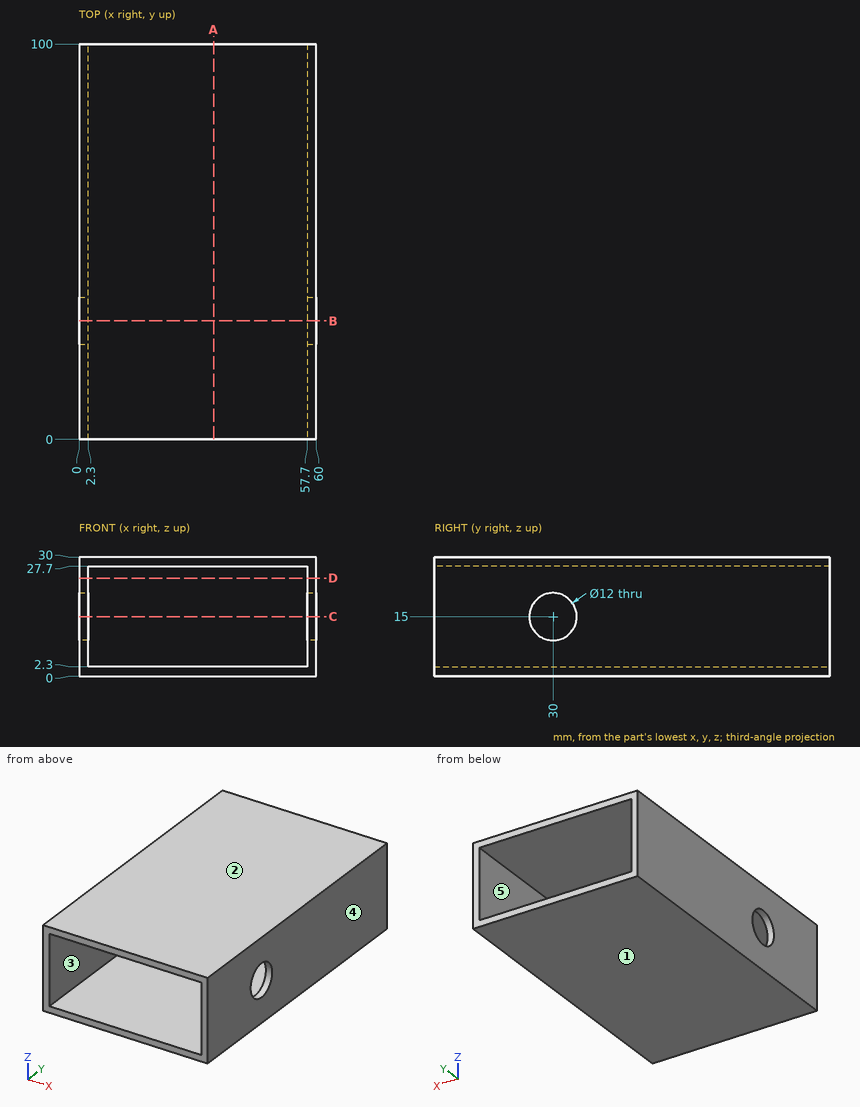
Check sheet for the drawn part. Datum: minimum x, y, z corner. Units: mm. A direction names the side the tool comes from. Coordinates: 2 decimals unless noted, no trailing zeros. Write each loop counter-clockwise with the first axis right and the second up, starting at its lowest first coordinate (ties: lowest second). Pieces come first, ordered by that corner, then holes. Notation, with made-up numbers: M 23,32.5 L 77,32.5 A33 cw 77,71.5 Z; hole C -21,27.5 d6. An arc over 180 degrees is marked long. One line per item, written item: value.
Item 1: Scan lines: line 1 along Z through (x, y) = (34, 49); line 2 along Y through (x, z) = (59, 15); line 3 along X through (y, z) = (8.5, 21.25). Record each from-to range of solid material in increasing order.
Check sheet entries:
line 1: z = 0 to 2.3, 27.7 to 30
line 2: y = 0 to 24, 36 to 100
line 3: x = 0 to 2.3, 57.7 to 60
Item 2: Access from +Z, -Z, +X, -X, +Y, -Y to the whole of each face (thin tool, end or side, straight path). Record for the marked faces 4 and 5.
Check sheet entries:
face 4: +Z, -Z, +X, +Y, -Y
face 5: +Y, -Y
Item 3: Section check B-B, the plane y = 30. Record the boundary of the cut face in (x, z), plus the area to 3 significant figures.
Check sheet entries:
outline: M 0,0 L 60,0 L 60,9 L 57.7,9 L 57.7,2.3 L 2.3,2.3 L 2.3,9 L 0,9 Z; M 0,21 L 2.3,21 L 2.3,27.7 L 57.7,27.7 L 57.7,21 L 60,21 L 60,30 L 0,30 Z
area: 338 mm^2
Item 4: Section check D-D, the plane z = 24.75. Record the boundary of the cut face in (x, y), plus the area to 3 significant figures.
Check sheet entries:
outline: M 0,0 L 2.3,0 L 2.3,100 L 0,100 Z; M 57.7,0 L 60,0 L 60,100 L 57.7,100 Z
area: 460 mm^2
Item 5: Mould release check, pull along Z, two halves, no side actions. Record for the marked faces 1, 2 and 3: pulls with the +Z half, pulls with the -Z half, needs draft (parallel to the pull), parting line crosses it, or undercut.
Check sheet entries:
face 1: pulls with the -Z half
face 2: pulls with the +Z half
face 3: undercut
Item 6: Section check A-A, the plane x = 34. Record the boundary of the cut face in (y, z), plus the area to 3 significant figures.
Check sheet entries:
outline: M 0,0 L 100,0 L 100,2.3 L 0,2.3 Z; M 0,27.7 L 100,27.7 L 100,30 L 0,30 Z
area: 460 mm^2
Item 7: Section check C-C, the plane z = 15. Record the boundary of the cut face in (x, y), plus the area to 3 significant figures.
Check sheet entries:
outline: M 0,0 L 2.3,0 L 2.3,24 L 0,24 Z; M 0,36 L 2.3,36 L 2.3,100 L 0,100 Z; M 57.7,0 L 60,0 L 60,24 L 57.7,24 Z; M 57.7,36 L 60,36 L 60,100 L 57.7,100 Z
area: 405 mm^2
